```python
from build123d import *

# Parameters (mm, degrees)
F0_R       = 12.1285
F1_DEPTH   = 21.4376
F2_SIZE2   = 1.7597636205
F2_SIZE    = 1.016
F2_2_SIZE2 = 1.7597636205
F2_2_SIZE  = 1.016
F3_R       = 9.8679
F4_DEPTH   = 4.318
F5_R       = 12.4714
F6_DEPTH   = 73.4314
F7_R       = 8.7122
F8_DEPTH   = 4.4196
F9_R       = 10.414
F10_DEPTH  = 21.59
F11_SIZE2  = 1.7597636205
F11_SIZE   = 1.016


with BuildPart() as f1:
    # F0 (on Front) → F1 (new body)
    with BuildSketch(Plane.XZ):
        Circle(F0_R)
    extrude(amount=F1_DEPTH)

    # F2
    f2_edges = [f1.edges().sort_by_distance(p)[0] for p in [
        (-12.1285, -21.4376, 0),
    ]]
    f2_side = f1.faces().sort_by_distance((0, -21.4376, 0))[0]
    chamfer(f2_edges, length=F2_SIZE, length2=F2_SIZE2, reference=f2_side)

    # F2#2
    f2_2_edges = [f1.edges().sort_by_distance(p)[0] for p in [
        (-12.1285, 0, 0),
    ]]
    f2_2_side = f1.faces().sort_by_distance((0, 0, 0))[0]
    chamfer(f2_2_edges, length=F2_2_SIZE, length2=F2_2_SIZE2, reference=f2_2_side)

    # F3 (on face) → F4 (join)
    with BuildSketch(Plane(origin=(0, 0, 0), x_dir=(-1, 0, 0), z_dir=(0, 1, 0))):
        Circle(F3_R)
    extrude(amount=F4_DEPTH)

    # F5 (on face) → F6 (join)
    with BuildSketch(Plane(origin=(0, 4.318, 0), x_dir=(-1, 0, 0), z_dir=(0, 1, 0))):
        Circle(F5_R)
    extrude(amount=F6_DEPTH)

    # F7 (on face) → F8 (join)
    with BuildSketch(Plane(origin=(0, 77.7494, 0), x_dir=(-1, 0, 0), z_dir=(0, 1, 0))):
        Circle(F7_R)
    extrude(amount=F8_DEPTH)

    # F9 (on face) → F10 (join)
    with BuildSketch(Plane(origin=(0, 82.169, 0), x_dir=(-1, 0, 0), z_dir=(0, 1, 0))):
        Circle(F9_R)
    extrude(amount=F10_DEPTH)

    # F11
    f11_edges = [f1.edges().sort_by_distance(p)[0] for p in [
        (10.414, 103.759, 0),
    ]]
    f11_side = f1.faces().sort_by_distance((0, 103.759, 0))[0]
    chamfer(f11_edges, length=F11_SIZE, length2=F11_SIZE2, reference=f11_side)


solid = f1.part
```
Model file for the job. Use its own axes, mm. A direction names the side the tool comes from. Round coordinates to 2 decimals unless told otherwise and drop trailing zeros. Order: outer loops, then holes, each group sorted by start corner. A loop starts at its lowest first (then second) coordinate and runs counter-clockwise, first axis right, second up. Notation, with made-up numbers: (-35, 56.25) -> (10, 56.25) arc R16 cw to (10, 82.25) -> close; hole circle Ø1 at (84, 84.5). An arc over 180 degrees is marked (long way). Use one line per item in the form item = value.
Item 1: Pull direction Y, two halves, no side cores. Call faces 1 (the face through (0, -21.438, 0)), 2 (the face through (0, 103.759, 0)), 3 (the face through (6.914, 79.928, -5.301)), 4 (the face through (-9.933, 91.945, 3.128)): released by +Y, released by -Y, zero draft, split by the parting line, or undercut.
Returned:
face_1 = released by -Y
face_2 = released by +Y
face_3 = undercut
face_4 = zero draft
Item 2: Flat gauge pins, fed straight in: pin 1 Ø2 at (x, y) = (4, 15.5) entering from -Z; pin 2 Ø3 at (y, z) = (71.5, -4.5) entering from -X; pin 3 Ø4 at (y, z) = (47.5, -2.5) entering from -X. Where does each tip first touch, or does it go through?
Returned:
pin_1 = -12.11
pin_2 = -12.11
pin_3 = -12.46
Item 3: Cut at D-D, the plane y = 54. Write the cut outline in (x, z).
Returned:
outline = circle Ø24.94 at (0, 0)
Item 4: Cut at A-A, the plane z = 0. Write the cut outline in (x, y).
Returned:
outline = (-12.47, 4.32) -> (-9.87, 4.32) -> (-9.87, 0) -> (-11.11, 0) -> (-12.13, -1.76) -> (-12.13, -19.68) -> (-11.11, -21.44) -> (11.11, -21.44) -> (12.13, -19.68) -> (12.13, -1.76) -> (11.11, 0) -> (9.87, 0) -> (9.87, 4.32) -> (12.47, 4.32) -> (12.47, 77.75) -> (8.71, 77.75) -> (8.71, 82.17) -> (10.41, 82.17) -> (10.41, 102) -> (9.4, 103.76) -> (-9.4, 103.76) -> (-10.41, 102) -> (-10.41, 82.17) -> (-8.71, 82.17) -> (-8.71, 77.75) -> (-12.47, 77.75) -> close
Item 5: Tool access for faces 5 (the face through (8.5, 77.749, -2.6)), 6 (the face through (11.57, -10.59, 3.64)), 7 (the face through (2.704, 40.52, -12.175)): list every direction of +Z, -Z, +X, -X, +Y, -Y with a clear straight run to the whole face (end or side of a thin tool).
Returned:
face_5 = none
face_6 = -Y
face_7 = +Y, -Y
Item 6: Drill centre lines: line 1 (Y direction, x = -2, z = -9); line 2 (Y direction, x = 9.5, z = -4.5); line 3 (Z direction, x = 0.5, y = 74). Where is each one in solid material? Low to high.
Returned:
line_1 = -21.44 to 77.75, 82.17 to 103.76
line_2 = -21.44 to 0, 4.32 to 77.75
line_3 = -12.46 to 12.46
Item 7: Cut at C-C, the plane y = -5.5. Write the cut outline in (x, z), and give its area (3 significant figures).
Returned:
outline = circle Ø24.26 at (0, 0)
area = 462 mm^2
Item 8: Cut at B-B, the plane x = 0. Write the cut outline in (y, z), and give its area (3 significant figures).
Returned:
outline = (-21.44, -11.11) -> (-19.68, -12.13) -> (-1.76, -12.13) -> (0, -11.11) -> (0, -9.87) -> (4.32, -9.87) -> (4.32, -12.47) -> (77.75, -12.47) -> (77.75, -8.71) -> (82.17, -8.71) -> (82.17, -10.41) -> (102, -10.41) -> (103.76, -9.4) -> (103.76, 9.4) -> (102, 10.41) -> (82.17, 10.41) -> (82.17, 8.71) -> (77.75, 8.71) -> (77.75, 12.47) -> (4.32, 12.47) -> (4.32, 9.87) -> (0, 9.87) -> (0, 11.11) -> (-1.76, 12.13) -> (-19.68, 12.13) -> (-21.44, 11.11) -> close
area = 2,960 mm^2
